Work out the finished part from the listing and answer in its coordinate system (mm). Face numbers are marked on the shaded views. Give positions to 0.01 mm unless a question says otherwise; leave off trailing zeros. Loops run counter-clockwise (first coordinate to the right, second up) from the corner with the lowest first, then second, coordinate; pieces in that order, holes last. Notation, with made-up numbers: (81.5, -39.5) - (86.5, -39.5) arc R14 ccw to (86.5, -16.5) - close; hole circle Ø11 at (84, -7). An arc over 180 degrees is marked (long way). Use one line per item in the form item = value. Start each with the question number.
from build123d import *

# Parameters (mm, degrees)
SKETCH1_R           = 63.5
BOSS_EXTRUDE1_DEPTH = 3.175
SKETCH2_R           = 60.325
SKETCH2_R_2         = 57.94375
BOSS_EXTRUDE2_DEPTH = 3.175
BOSS_EXTRUDE3_DEPTH = 127
FILLET1_R           = 12.7


with BuildPart() as part:
    # Sketch1 → Boss-Extrude1 (new body)
    with BuildSketch(Plane(origin=(0, 0, 0), x_dir=(1, 0, 0), z_dir=(0, 1, 0))):
        Circle(SKETCH1_R)
    extrude(amount=BOSS_EXTRUDE1_DEPTH)

    # Sketch2 → Boss-Extrude2 (add)
    with BuildSketch(Plane(origin=(0, 3.175, 0), x_dir=(1, 0, 0), z_dir=(0, 1, 0))):
        Circle(SKETCH2_R)
        Circle(SKETCH2_R_2, mode=Mode.SUBTRACT)
    extrude(amount=BOSS_EXTRUDE2_DEPTH)

    # Sketch3 → Boss-Extrude3 (add)
    with BuildSketch(Plane.XZ):
        with BuildLine():
            Line((-0.79375, 63.495038869), (-0.79375, 0.165767528))
            add(Edge.make_bspline(
                [(-0.79375, 0.165767528), (-5.19662587, 0.926394102), (-12.028294814, 1.162164763), (-21.507708178, -0.414484498), (-28.959628823, -2.648391287), (-36.549761029, -5.897616417), (-42.990474773, -9.452796753), (-48.210003566, -12.80329328), (-52.163993282, -15.574258653), (-55.991469214, -18.475868316), (-58.550879749, -20.554822593), (-59.733413602, -21.544588636)],
                knots=[0.02237317, 0.02237317, 0.02237317, 0.02237317, 0.257875777, 0.382709096, 0.507542415, 0.632375733, 0.757209052, 0.819625711, 0.882042371, 0.94445903, 1.000095669, 1.000095669, 1.000095669, 1.000095669], degree=3))
            ThreePointArc((-59.733413602, -21.544588636), (-59.442577848, -22.334501085), (-59.141296843, -23.120488916))
            add(Edge.make_bspline(
                [(0, -1.594817249), (-4.497680515, -0.712511058), (-11.342121161, -0.373927815), (-20.797455162, -1.88480643), (-28.048219709, -4.011073511), (-35.464551173, -7.138170569), (-41.780862519, -10.584133838), (-46.914506534, -13.847671974), (-50.8035363, -16.548272657), (-54.079771454, -19.012705913), (-56.859334031, -21.22174097), (-58.343356695, -22.447695352), (-59.141296843, -23.120488916)],
                knots=[0.002745404, 0.002745404, 0.002745404, 0.002745404, 0.252059053, 0.376715878, 0.501372702, 0.626029527, 0.750686351, 0.813014763, 0.875343176, 0.937671588, 0.968835794, 1.006875689, 1.006875689, 1.006875689, 1.006875689], degree=3))
            add(Edge.make_bspline(
                [(59.141296843, -23.120488916), (58.343356695, -22.447695352), (56.859334031, -21.22174097), (54.079771454, -19.012705913), (50.8035363, -16.548272657), (46.914506534, -13.847671974), (41.780862519, -10.584133838), (35.464551173, -7.138170569), (28.048219709, -4.011073511), (20.797455162, -1.88480643), (11.342121161, -0.373927815), (4.497680515, -0.712511058), (0, -1.594817249)],
                knots=[-0.004130285, -0.004130285, -0.004130285, -0.004130285, 0.03390961, 0.065073816, 0.127402229, 0.189730641, 0.252059053, 0.376715878, 0.501372702, 0.626029527, 0.750686351, 1, 1, 1, 1], degree=3))
            ThreePointArc((59.141296843, -23.120488916), (59.442577848, -22.334501085), (59.733413602, -21.544588636))
            add(Edge.make_bspline(
                [(59.733413602, -21.544588636), (58.550879749, -20.554822593), (55.991469214, -18.475868316), (52.163993282, -15.574258653), (48.210003566, -12.80329328), (42.990474773, -9.452796753), (36.549761029, -5.897616417), (28.959628823, -2.648391287), (21.507708178, -0.414484498), (12.028294814, 1.162164763), (5.19662587, 0.926394102), (0.79375, 0.165767528)],
                knots=[0.002649735, 0.002649735, 0.002649735, 0.002649735, 0.058286374, 0.120703033, 0.183119693, 0.245536352, 0.370369671, 0.495202989, 0.620036308, 0.744869627, 0.980372234, 0.980372234, 0.980372234, 0.980372234], degree=3))
            Line((0.79375, 0.165767528), (0.79375, 63.495038869))
            ThreePointArc((0.79375, 63.495038869), (0, 63.5), (-0.79375, 63.495038869))
        make_face()
    extrude(amount=BOSS_EXTRUDE3_DEPTH)

    # Fillet1
    fillet1_edges = [part.edges().sort_by_distance(p)[0] for p in [
        (0.79375, -63.5, 0.165767528),
        (-0.79375, -63.5, 0.165767528),
    ]]
    fillet(fillet1_edges, radius=FILLET1_R)


solid = part.part
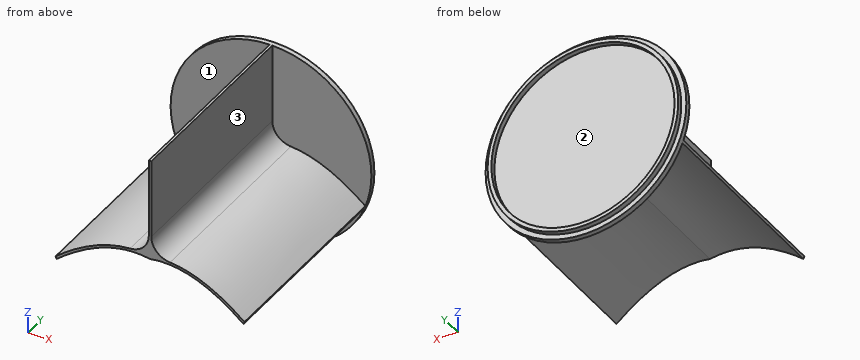
1) A cutting plane is placed at B-B (z = -51). Give the vertices of the cut face in (x, y) (3 decimals), plus the area to 3 significant figures.
2) A cutting plane is placed at A-A (z = -27.5). Give the vertices of the cut face in (x, y) (3 decimals), plus the area to 3 significant figures.
3) Find the intervals of material crossed by probe 1 along Z at (x, y) = (0, 4) (3 decimals); probe 2 along X at (y, z) = (-76, 12.5), in increasing order.
4) Flat-ended cylindrical pins translate along their axes: pin 1 Ø3 at (y, z) = (-7.5, 31) entering from -X; pin 2 Ø5 at (x, z) = (27.5, -37) entering from -Y; pin 3 Ø2 at (x, y) = (39, -11.5) entering from +Z. Find the tip coordinate at first contact, or state that the pin passes through.
5) Determine the mould class of the marked faces 1, 2 and 3 for opening direction X: released by +X, released by -X, zero draft, split by the parting line, or undercut.
Answer sheet:
q1.outline = (-37.832, 0) - (37.832, 0) - (37.832, 3.175) - (32.22, 3.175) - (32.22, 6.35) - (27.504, 6.35) - (27.504, 3.175) - (-27.504, 3.175) - (-27.504, 6.35) - (-32.22, 6.35) - (-32.22, 3.175) - (-37.832, 3.175) - close
q1.area = 270 mm²
q2.outline = (-57.236, 0) - (57.236, 0) - (57.236, 3.175) - (53.692, 3.175) - (53.692, 6.35) - (51.002, 6.35) - (51.002, 3.175) - (-51.002, 3.175) - (-51.002, 6.35) - (-53.692, 6.35) - (-53.692, 3.175) - (-57.236, 3.175) - close
q2.area = 381 mm²
q3.probe_1 = -60.325 to -57.944, 57.944 to 60.325
q3.probe_2 = -0.83 to 0.83
q4.pin_1 = -0.79
q4.pin_2 = 0
q4.pin_3 = -6.78
q5.face_1 = zero draft
q5.face_2 = undercut
q5.face_3 = released by +X
